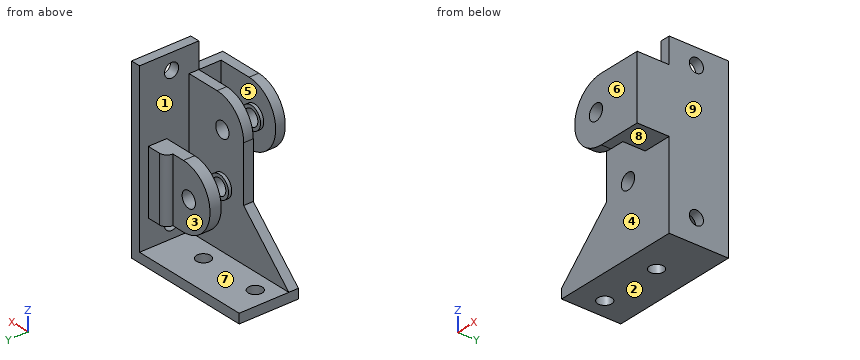
from build123d import *

# Parameters (mm, degrees)
BOSS_EXTRUDE1_DEPTH = 18.5
BOSS_EXTRUDE2_DEPTH = 3
BOSS_EXTRUDE3_START = 7
BOSS_EXTRUDE3_DEPTH = 3.5
SKETCH4_W           = 6.5
SKETCH4_H           = 2.25
BOSS_EXTRUDE4_DEPTH = 20
FILLET1_R           = 2.25
BOSS_EXTRUDE5_DEPTH = 7
BOSS_EXTRUDE6_START = 3
BOSS_EXTRUDE6_DEPTH = 3
SKETCH7_R           = 2.5
CUT_EXTRUDE1_DEPTH  = 73.232264259
SKETCH8_R           = 2.2
CUT_EXTRUDE2_DEPTH  = 71.763691255
CUT_EXTRUDE3_REACH  = 72.764
SKETCH9_R           = 2.2
BOSS_EXTRUDE7_REACH = 74.907
SKETCH10_R          = 3.5
SKETCH10_R_2        = 2.5
BOSS_EXTRUDE8_REACH = 72.039
SKETCH11_R          = 3.5
SKETCH11_R_2        = 2.5
CUT_EXTRUDE4_REACH  = 66.742
SKETCH12_W          = 7
SKETCH12_H          = 5


with BuildPart() as part:
    # Sketch1 → Boss-Extrude1 (new body)
    with BuildSketch(Plane(origin=(0, 0, 0), x_dir=(1, 0, 0), z_dir=(0, 1, 0))):
        Polygon((-40.5, 0), (0, 0), (0, -55), (-3, -55), (-3, -3), (-40.5, -3), align=None)
    extrude(amount=BOSS_EXTRUDE1_DEPTH)

    # Sketch2 → Boss-Extrude2 (add)
    with BuildSketch(Plane.XZ):
        with BuildLine():
            Line((-40.5, 3), (-23.5, 19.5))
            Line((-23.5, 19.5), (-23.5, 37))
            ThreePointArc((-23.5, 37), (-20.571067812, 44.071067812), (-13.5, 47))
            Line((-13.5, 47), (-3, 47))
            Line((-3, 47), (-3, 3))
            Line((-3, 3), (-40.5, 3))
        make_face()
    extrude(amount=-BOSS_EXTRUDE2_DEPTH)

    # Sketch3 → Boss-Extrude3 (add)
    with BuildSketch(Plane(origin=(0, 3, 0), x_dir=(1, 0, 0), z_dir=(0, 1, 0)).offset(BOSS_EXTRUDE3_START)):
        with BuildLine():
            Line((-3, -31.5), (-13.5, -31.5))
            ThreePointArc((-13.5, -31.5), (-23.5, -21.5), (-13.5, -11.5))
            Line((-13.5, -11.5), (-3, -11.5))
            Line((-3, -11.5), (-3, -31.5))
        make_face()
    extrude(amount=BOSS_EXTRUDE3_DEPTH)

    # Sketch4 → Boss-Extrude4 (add)
    with BuildSketch(Plane.XY.offset(31.5)):
        with Locations((-6.25, 14.625)):
            Rectangle(SKETCH4_W, SKETCH4_H)
    extrude(amount=-BOSS_EXTRUDE4_DEPTH)

    # Fillet1
    fillet1_edges = [part.edges().sort_by_distance(p)[0] for p in [
        (-9.5, 15.75, 21.5),
    ]]
    fillet(fillet1_edges, radius=FILLET1_R - 0.0001)  # a hair under: the kernel refuses the full size

    # Sketch5 → Boss-Extrude5 (add)
    with BuildSketch(Plane.XZ):
        Polygon((0, 47), (0, 27), (-9, 27), (-9, 29), (-3, 29), (-3, 47), align=None)
    extrude(amount=BOSS_EXTRUDE5_DEPTH)

    # Sketch6 → Boss-Extrude6 (add)
    with BuildSketch(Plane.XZ.offset(7).offset(BOSS_EXTRUDE6_START)):
        with BuildLine():
            Line((0, 27), (0, 47))
            Line((0, 47), (-13.5, 47))
            ThreePointArc((-13.5, 47), (-23.5, 37), (-13.5, 27))
            Line((-13.5, 27), (0, 27))
        make_face()
    extrude(amount=-BOSS_EXTRUDE6_DEPTH)

    # Sketch7 → Cut-Extrude1 (cut, through all)
    with BuildSketch(Plane(origin=(0, 13.5, 0), x_dir=(1, 0, 0), z_dir=(0, 1, 0))):
        with Locations(Location((-15.5, -21.5, 0), (0, 0, 270))):
            Circle(SKETCH7_R)
        with Locations(Location((-15.5, -37, 0), (0, 0, 270))):
            Circle(SKETCH7_R)
    extrude(amount=-CUT_EXTRUDE1_DEPTH, mode=Mode.SUBTRACT)

    # Sketch8 → Cut-Extrude2 (cut, through all)
    with BuildSketch(Plane(origin=(0, 0, 0), x_dir=(0, 0, -1), z_dir=(1, 0, 0))):
        with Locations((-50, 8.5)):
            Circle(SKETCH8_R)
        with Locations((-7.5, 8.5)):
            Circle(SKETCH8_R)
    extrude(amount=-CUT_EXTRUDE2_DEPTH, mode=Mode.SUBTRACT)

    # Sketch9 → Cut-Extrude3 (cut, up to next)
    with BuildSketch(Plane(origin=(0, 0, 0), x_dir=(-1, 0, 0), z_dir=(0, 0, -1)), mode=Mode.PRIVATE) as cut_extrude3_sk1:
        with Locations((15, 8.5)):
            Circle(SKETCH9_R)
    cut_extrude3_tool1 = extrude(cut_extrude3_sk1.sketch, amount=-CUT_EXTRUDE3_REACH, mode=Mode.PRIVATE) & part.part
    # Sketch9 → Cut-Extrude3 (cut, up to next)
    with BuildSketch(Plane(origin=(0, 0, 0), x_dir=(-1, 0, 0), z_dir=(0, 0, -1)), mode=Mode.PRIVATE) as cut_extrude3_sk2:
        with Locations((34.5, 8.5)):
            Circle(SKETCH9_R)
    cut_extrude3_tool2 = extrude(cut_extrude3_sk2.sketch, amount=-CUT_EXTRUDE3_REACH, mode=Mode.PRIVATE) & part.part
    add(cut_extrude3_tool1.solids().sort_by_distance((-15, 8.5, 0))[0], mode=Mode.SUBTRACT)
    add(cut_extrude3_tool2.solids().sort_by_distance((-34.5, 8.5, 0))[0], mode=Mode.SUBTRACT)

    # Sketch10 → Boss-Extrude7 (add, up to next)
    with BuildSketch(Plane(origin=(0, -7, 0), x_dir=(1, 0, 0), z_dir=(0, 1, 0)), mode=Mode.PRIVATE) as boss_extrude7_sk1:
        with Locations(Location((-15.5, -37, 0), (0, 0, 90))):
            Circle(SKETCH10_R)
        with Locations(Location((-15.5, -37, 0), (0, 0, 270))):
            Circle(SKETCH10_R_2, mode=Mode.SUBTRACT)
    boss_extrude7_tool1 = extrude(boss_extrude7_sk1.sketch, amount=BOSS_EXTRUDE7_REACH, mode=Mode.PRIVATE) - part.part
    add(boss_extrude7_tool1.solids().sort_by_distance((-15.5, -7, 40.401005))[0])

    # Sketch11 → Boss-Extrude8 (add, up to next)
    with BuildSketch(Plane(origin=(0, 3, 0), x_dir=(1, 0, 0), z_dir=(0, 1, 0)), mode=Mode.PRIVATE) as boss_extrude8_sk1:
        with Locations(Location((-15.5, -21.5, 0), (0, 0, 90))):
            Circle(SKETCH11_R)
        with Locations(Location((-15.5, -21.5, 0), (0, 0, 270))):
            Circle(SKETCH11_R_2, mode=Mode.SUBTRACT)
    boss_extrude8_tool1 = extrude(boss_extrude8_sk1.sketch, amount=BOSS_EXTRUDE8_REACH, mode=Mode.PRIVATE) - part.part
    add(boss_extrude8_tool1.solids().sort_by_distance((-15.5, 3, 24.901005))[0])

    # Cut-Extrude4: up to this face of the body (flat: up to its plane)
    cut_extrude4_end = Plane(part.part.faces().sort_by_distance((-21.584376674, 10.874217494, 3))[0])
    # Sketch12 → Cut-Extrude4 (cut, up to the picked face)
    with BuildSketch(Plane.XY.offset(47), mode=Mode.PRIVATE) as cut_extrude4_sk1:
        with Locations((-15.5, -3.5)):
            Rectangle(SKETCH12_W, SKETCH12_H)
    cut_extrude4_tool1 = split(extrude(cut_extrude4_sk1.sketch, amount=-CUT_EXTRUDE4_REACH, mode=Mode.PRIVATE), bisect_by=cut_extrude4_end, keep=Keep.BOTH, mode=Mode.PRIVATE)
    # Sketch12 → Cut-Extrude4 (cut, up to the picked face)
    with BuildSketch(Plane.XY.offset(47), mode=Mode.PRIVATE) as cut_extrude4_sk2:
        with Locations((-15.5, 6.5)):
            Rectangle(SKETCH12_W, SKETCH12_H)
    cut_extrude4_tool2 = split(extrude(cut_extrude4_sk2.sketch, amount=-CUT_EXTRUDE4_REACH, mode=Mode.PRIVATE), bisect_by=cut_extrude4_end, keep=Keep.BOTH, mode=Mode.PRIVATE)
    add(cut_extrude4_tool1.solids().sort_by(Axis((-15.5, -3.5, 47), (0, 0, -1)))[0], mode=Mode.SUBTRACT)
    add(cut_extrude4_tool2.solids().sort_by(Axis((-15.5, 6.5, 47), (0, 0, -1)))[0], mode=Mode.SUBTRACT)


solid = part.part
The model under review builds one solid part; all positions refer to its coordinate system, in mm. Face numbers are marked on the shaded views. A direction names the side the tool comes from. Coordinates: 2 decimals unless noted, no trailing zeros. Loops run counter-clockwise (first coordinate to the right, second up) from the corner with the lowest first, then second, coordinate; pieces in that order, holes last. Notation, with made-up numbers: M 78,30.5 L 82,30.5 A32 cw 82,61.5 Z; hole C 17.5,-11.5 d5. An arc over 180 degrees is marked long. Put each result on its own line as item: value. Start each with the question number.
Q1. Wall thickness on line 1 (Z direction, x = -7.5, y = 12.5); line 2 (Y direction, x = -6, z = 45); line 3 (X direction, y = 1.65, z = 21.5): over which ranges is each line inside the solid? List them lowest first.
Q2. Add section B-B (x = -10.5). Write out the cut boundary in (y, z).
Q3. Add section A-A (z = 50). Write out the cut boundary in (x, y).
Q4. Add section C-C (z = 36). Write out the cut boundary in (x, y), and give its area (3 significant figures).
Q5. Add section D-D (y = -4). Write out the cut boundary in (x, z).
Q6. The part is to be moulded in two halves that separate along Y. For the marked faces 1, 2, 3 and 4, say which applies: +Y half, -Y half, draft (parallel to the pull), parting line (faces both ways), or undercut.
Q7. Clearance check with flat-ended pins moving along their axes: pin 1 (1.5 mm diameter, centred on y = 2, z = 30.5, fed in from -X); pin 2 (6 mm diameter, centred on x = -11, y = -4.5, fed in from +Z); pin 3 (12 mm diameter, centred on x = -20.5, z = 25, fed in from +Y); pin 4 (2.5 mm diameter, centred on x = -34.5, y = 8.5, fed in from +Z). State where each tip first meets the part, or that it passes through.
Q8. For the marked faces 5, 6, 7, 8 and 9, list the 3-axis set-ups (+Z, -Z, +X, -X, +Y, -Y) from which the entire face can be reached by the end or side of a thin tool; tool diameter is ignored.
Answers:
1. line 1: z = 0 to 3, 11.5 to 31.5
1. line 2: y = -10 to -7, 0 to 3
1. line 3: x = -23.5 to -18, -13 to 0
2. outline: M -10,27 L -7,27 L -7,47 L -10,47 Z; M 0,0 L 18.5,0 L 18.5,3 L 3,3 L 3,47 L 0,47 Z; M 10,11.5 L 13.5,11.5 L 13.5,31.5 L 10,31.5 Z
3. outline: M -3,0 L 0,0 L 0,6.3 L -3,6.3 Z; M -3,10.7 L 0,10.7 L 0,18.5 L -3,18.5 Z
4. outline: M -23.5,0 L -18.85,0 L -18.85,-1 L -17.79,-1 L -17.79,3 L -23.5,3 Z; M -23.45,-10 L -17.79,-10 L -17.79,-6 L -18.85,-6 L -18.85,-7 L -23.45,-7 Z; M -13.21,-10 L 0,-10 L 0,18.5 L -3,18.5 L -3,3 L -13.21,3 L -13.21,-1 L -12.15,-1 L -12.15,0 L -3,0 L -3,-7 L -12.15,-7 L -12.15,-6 L -13.21,-6 Z
4. area: 185 mm^2
5. outline: M -9,27 L 0,27 L 0,47 L -3,47 L -3,29 L -9,29 Z
6. face 1: undercut
6. face 2: draft
6. face 3: +Y half
6. face 4: undercut
7. pin 1: stops at x = -23.5
7. pin 2: stops at z = 47
7. pin 3: stops at y = 13.5
7. pin 4: passes through
8. face 5: none
8. face 6: +Z, -Z, +X, -X, -Y
8. face 7: -X, +Y
8. face 8: -Z, +X, -X, -Y
8. face 9: +Z, -Z, +X, +Y, -Y
